Can you work these out from the drawing? Everything is in mm from the part's minimum corner. A direction names the side the tool comes from. Round coordinates to 2 decimals unless told otherwise and drop trailing zeros. Write each loop counter-clockwise with the first axis right and the second up, starting at its lowest first coordinate (ties: lowest second). Pieces come first, ordered by that corner, then holes.
Q1. If we section it at B-B (y = 10.75): Please give me the cut outline in (x, z).
Q2. We'd pull the mould along Y, two halves only. Please class the marked faces 1, 2, 3 and 4: +Y half, -Y half, draft (parallel to the pull), parting line (faces both ways), or undercut.
Q3. If we section it at C-C (x = 8): Please give me the cut outline in (y, z) (1 decimal), plus the area to 3 significant figures.
Q4. For the marked faces 5 and 6, which set-ups out of +Z, -Z, +X, -X, +Y, -Y let a thin tool reach every point of the face, with its end or its side?
Q5. If we section it at A-A (z = 2.25): Please give me the cut outline in (x, y), plus the area to 3 significant figures.
Q6. Please list where these lines run through material, in increasing order: line 1 along X through (y, z) = (10, 1.5) (1 decimal); line 2 along Y through (x, z) = (24.5, 6.25); line 3 along Y through (x, z) = (6, 0.5).
Q7. I'm going to push flat-ended pins straight in: pin 1 Ø3.5 at (x, z) = (8.5, 2.5) entering from +Y; pin 2 Ø3 at (x, z) = (7, 6) entering from -Y; pin 3 Ø1.5 at (x, y) = (10, 6.5) entering from +Z; pin 4 Ø3.5 at (x, z) = (9, 3) entering from -Y. Where does each tip first touch, or does it pass through?
Q8. If we section it at D-D (x = 14.25): Please give me the cut outline in (y, z).
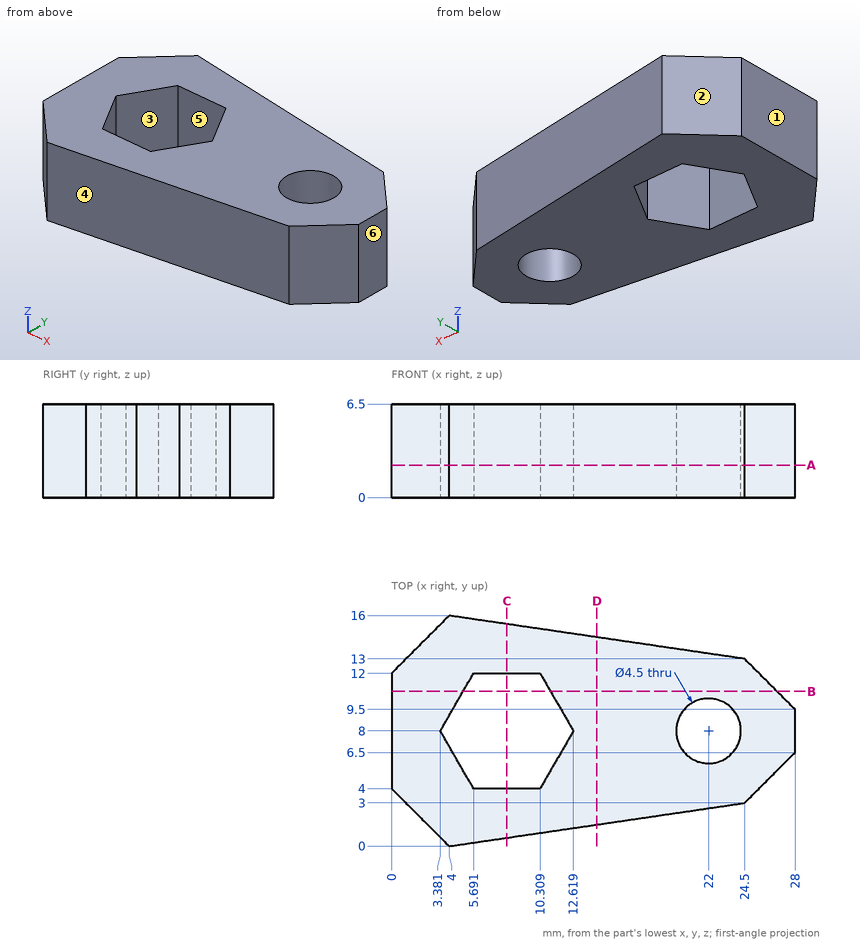
A:
1. outline: (0, 0) - (4.97, 0) - (4.97, 6.5) - (0, 6.5) - close; (11.03, 0) - (26.75, 0) - (26.75, 6.5) - (11.03, 6.5) - close
2. face 1: draft
2. face 2: +Y half
2. face 3: undercut
2. face 4: -Y half
3. outline: (0.6, 0) - (4, 0) - (4, 6.5) - (0.6, 6.5) - close; (12, 0) - (15.4, 0) - (15.4, 6.5) - (12, 6.5) - close
3. area: 44.4 mm2
4. face 5: +Z, -Z
4. face 6: +Z, -Z, +X, +Y, -Y
5. outline: (0, 4) - (4, 0) - (24.5, 3) - (28, 6.5) - (28, 9.5) - (24.5, 13) - (4, 16) - (0, 12) - close; hole (3.38, 8) - (5.69, 4) - (10.31, 4) - (12.62, 8) - (10.31, 12) - (5.69, 12) - close; hole circle Ø4.5 at (22, 8)
5. area: 266 mm2
6. line 1: x = 0 to 4.5, 11.5 to 21, 23 to 27.5
6. line 2: y = 3 to 13
6. line 3: y = 0.29 to 4, 12 to 15.71
7. pin 1: stops at y = 15.6
7. pin 2: stops at y = 0.22
7. pin 3: passes through
7. pin 4: stops at y = 0.48
8. outline: (1.5, 0) - (14.5, 0) - (14.5, 6.5) - (1.5, 6.5) - close
